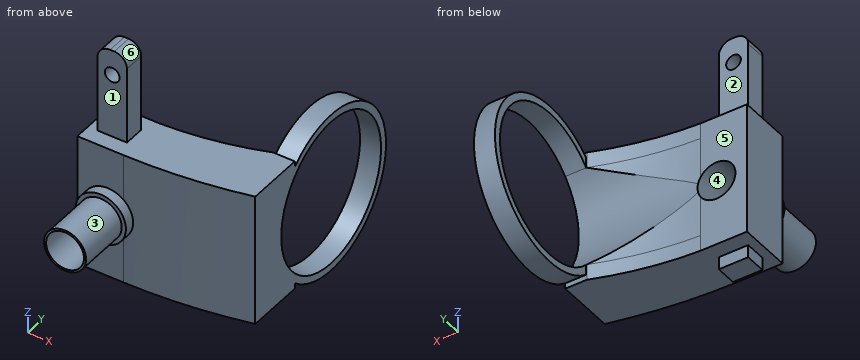
from build123d import *

# Parameters (mm, degrees)
BOSS_EXTRUDE1_DEPTH       = 48
SKETCH2_W                 = 14
SKETCH2_H                 = 10
BOSS_EXTRUDE2_DEPTH       = 50
CUT_EXTRUDE1_DEPTH        = 98
M8X1_0_TAPPED_HOLE1_D     = 7
M8X1_0_TAPPED_HOLE1_DEPTH = 10
M8X1_0_TAPPED_HOLE1_TIP   = 2.103012167
FILLET1_R                 = 6
SKETCH7_R                 = 38.5
SKETCH7_R_2               = 35
BOSS_EXTRUDE3_DEPTH       = 10
SKETCH8_R                 = 35
CUT_EXTRUDE2_DEPTH        = 90
BOSS_EXTRUDE4_DEPTH       = 5
BOSS_EXTRUDE4_DEPTH_BACK  = 10
SKETCH10_R                = 12
SKETCH10_R_2              = 9
BOSS_EXTRUDE5_START       = 25
SKETCH11_R                = 10
SKETCH11_R_2              = 9
BOSS_EXTRUDE5_DEPTH       = 25
SKETCH12_R                = 9
CUT_EXTRUDE3_DEPTH        = 42
BOSS_EXTRUDE6_DEPTH       = 7.5
BOSS_EXTRUDE7_START       = 7.5
BOSS_EXTRUDE7_DEPTH       = 7.5


with BuildPart() as part:
    # Sketch1 → Boss-Extrude1 (new body)
    with BuildSketch(Plane.XY):
        with BuildLine():
            Line((0, 0), (0, 25.00039893))
            Line((0, 25.00039893), (22, 25.00039893))
            ThreePointArc((22, 25.00039893), (51.667114877, 29.062120939), (80, 38.751440389))
            Line((80, 38.751440389), (80, 6.798665084))
            ThreePointArc((80, 6.798665084), (51.198552391, 1.705464917), (22, 0))
            Line((22, 0), (0, 0))
        make_face()
    extrude(amount=BOSS_EXTRUDE1_DEPTH)

    # Sketch2 → Boss-Extrude2 (add)
    with BuildSketch(Plane.XY.offset(48)):
        with Locations((11.5, 12.5)):
            Rectangle(SKETCH2_W, SKETCH2_H)
    boss_extrude2 = extrude(amount=BOSS_EXTRUDE2_DEPTH)

    # Mirror1: Boss-Extrude2 across plane
    add(boss_extrude2.mirror(Plane.XY.offset(24)))

    # Sketch3 → Cut-Extrude1 (cut)
    with BuildSketch(Plane(origin=(0, 0, 0), x_dir=(1, 0, 0), z_dir=(0, 1, 0))):
        Polygon((32.759036304, 13.5), (11.5, 13.5), (-23.123003772, 13.5), (-23.123003772, 84.867154232), (32.759036304, 84.867154232), align=None)
    extrude(amount=CUT_EXTRUDE1_DEPTH, mode=Mode.SUBTRACT)

    # M8x1.0 Tapped Hole1
    with Locations(Plane(origin=(11.5, 17.5, 86), x_dir=(0, 0, 1), z_dir=(0, 1, 0))):
        with Locations((0, 0)):
            Hole(M8X1_0_TAPPED_HOLE1_D / 2, depth=M8X1_0_TAPPED_HOLE1_DEPTH)
            with Locations((0, 0, -(M8X1_0_TAPPED_HOLE1_DEPTH + M8X1_0_TAPPED_HOLE1_TIP / 2))):  # 118° drill point
                Cone(0, M8X1_0_TAPPED_HOLE1_D / 2, M8X1_0_TAPPED_HOLE1_TIP, mode=Mode.SUBTRACT)

    # Fillet1
    fillet1_edges = [part.edges().sort_by_distance(p)[0] for p in [
        (18.5, 12.5, 98),
        (4.5, 12.5, 98),
    ]]
    fillet(fillet1_edges, radius=FILLET1_R)

    # Sketch7 → Boss-Extrude3 (add)
    with BuildSketch(Plane.ZY.offset(-80)):
        with Locations((24, 60.00039893)):
            Circle(SKETCH7_R)
        with Locations((24, 60.00039893)):
            Circle(SKETCH7_R_2, mode=Mode.SUBTRACT)
    extrude(amount=BOSS_EXTRUDE3_DEPTH)

    # Sketch8 → Cut-Extrude2 (cut)
    with BuildSketch(Plane.ZY.offset(-80)):
        with Locations(Location((24, 60.00039893, 0), (0, 0, 226.708192407))):
            Circle(SKETCH8_R)
    extrude(amount=CUT_EXTRUDE2_DEPTH, mode=Mode.SUBTRACT)

    # Sketch10 → Boss-Extrude4 (add, two sides: drawn at the far end of the back side and taken through both)
    with BuildSketch(Plane.XZ.offset(-BOSS_EXTRUDE4_DEPTH_BACK)):
        with Locations((14.5, 24)):
            Circle(SKETCH10_R)
        with Locations((14.5, 24)):
            Circle(SKETCH10_R_2, mode=Mode.SUBTRACT)
    extrude(amount=BOSS_EXTRUDE4_DEPTH + BOSS_EXTRUDE4_DEPTH_BACK)

    # Sketch11 → Boss-Extrude5 (add)
    with BuildSketch(Plane.XZ.offset(5).offset(BOSS_EXTRUDE5_START)):
        with Locations((14.5, 24)):
            Circle(SKETCH11_R)
        with Locations((14.5, 24)):
            Circle(SKETCH11_R_2, mode=Mode.SUBTRACT)
    extrude(amount=-BOSS_EXTRUDE5_DEPTH)

    # Sketch12 → Cut-Extrude3 (cut)
    with BuildSketch(Plane(origin=(0, 0, 0), x_dir=(-1, 0, 0), z_dir=(0, -1, 0))):
        with Locations(Location((-14.5, -24, 0), (0, 0, 180))):
            Circle(SKETCH12_R)
    extrude(amount=-CUT_EXTRUDE3_DEPTH, mode=Mode.SUBTRACT)

    # Sketch13 → Boss-Extrude6 (add)
    with BuildSketch(Plane.XY.offset(48)):
        with BuildLine():
            Line((0, 25.00039893), (0, 0))
            Line((0, 0), (22, 0))
            ThreePointArc((22, 0), (51.198552391, 1.705464917), (80, 6.798665084))
            Line((80, 6.798665084), (80, 29.896412483))
            Line((80, 29.896412483), (80, 34.524920524))
            Line((80, 34.524920524), (70, 34.524920524))
            Line((70, 34.524920524), (69.729925021, 34.524920524))
            ThreePointArc((69.729925021, 34.524920524), (46.24106465, 27.877911315), (22, 25.00039893))
            Line((22, 25.00039893), (0, 25.00039893))
        make_face()
    extrude(amount=BOSS_EXTRUDE6_DEPTH)

    # Sketch14 → Boss-Extrude7 (add)
    with BuildSketch(Plane(origin=(0, 0, 0), x_dir=(-1, 0, 0), z_dir=(0, 0, -1)).offset(BOSS_EXTRUDE7_START)):
        with BuildLine():
            Line((-80, 29.896412483), (-80, 6.798665084))
            ThreePointArc((-80, 6.798665084), (-51.198552391, 1.705464917), (-22, 0))
            Line((-22, 0), (0, 0))
            Line((0, 0), (0, 25.00039893))
            Line((0, 25.00039893), (-22, 25.00039893))
            ThreePointArc((-22, 25.00039893), (-46.24106465, 27.877911315), (-69.729925021, 34.524920524))
            Line((-69.729925021, 34.524920524), (-70, 34.524920524))
            Line((-70, 34.524920524), (-80, 34.524920524))
            Line((-80, 34.524920524), (-80, 29.896412483))
        make_face()
    extrude(amount=-BOSS_EXTRUDE7_DEPTH)


solid = part.part
Geometry: final body of the model. Coordinates: model frame, mm. Face numbers are marked on the shaded views. A direction names the side the tool comes from. Give positions to 0.01 mm unless a question says otherwise; leave off trailing zeros. Write each loop counter-clockwise with the first axis right and the second up, starting at its lowest first coordinate (ties: lowest second). Pieces come first, ordered by that corner, then holes. Notation, with made-up numbers: (79, 28) -> (87, 28) arc R27 ccw to (87, 56) -> close; hole circle Ø9 at (82, -24). An arc over 180 degrees is marked (long way). Answer as a JSON object with one key per item and string values.
1. Mould query, pull axis X, two halves, no side actions, for the marked faces 4, 5 and 6. Classes: pulls with the +X half, pulls with the -X half, needs draft (parallel to the pull), parting line crosses it, or undercut.
Ans:
{"face 4": "undercut", "face 5": "needs draft", "face 6": "pulls with the +X half"}
2. Access query for the marked faces 1, 2 and 3. Directions: +Z, -Z, +X, -X, +Y, -Y. A direction counts if a zero-diameter tool reaches every point of the face in a straight line with its end or side. Return the directions, or none.
Ans:
{"face 1": "+Z, +X, -X, -Y", "face 2": "+Z, +X, -X, +Y", "face 3": "-Y"}
3. Cut plane A-A on z = 24. Output: boundary loops of the cut face in (x, y).
Ans:
{"outline": "(0, 0) -> (2.5, 0) -> (2.5, -5) -> (4.5, -5) -> (4.5, -30) -> (5.5, -30) -> (5.5, 25) -> (0, 25) -> close; (23.5, -30) -> (24.5, -30) -> (24.5, -5) -> (26.5, -5) -> (26.5, 0.04) arc R250.8 ccw to (80, 6.8) -> (80, 25) -> (23.5, 25) -> close; (70, 95) -> (80, 95) -> (80, 98.5) -> (70, 98.5) -> close"}
4. Cut plane D-D on x = 36. Output: boundary loops of the cut face in (y, z).
Ans:
{"outline": "(0.39, -7.5) -> (26.19, -7.5) -> (26.19, 14.96) arc R35 cw to (26.19, 33.04) -> (26.19, 55.5) -> (0.39, 55.5) -> close"}
5. Cut plane C-C on y = 11.5. Output: boundary loops of the cut face in (x, z).
Ans:
{"outline": "(0, -7.5) -> (4.5, -7.5) -> (4.5, -13.5) -> (18.5, -13.5) -> (18.5, -7.5) -> (80, -7.5) -> (80, 55.5) -> (18.5, 55.5) -> (18.5, 92) arc R6 ccw to (12.5, 98) -> (10.5, 98) arc R6 ccw to (4.5, 92) -> (4.5, 55.5) -> (0, 55.5) -> close; hole circle Ø18 at (14.5, 24); hole circle Ø7 at (11.5, 86)"}
6. Ray query, probe 1 along Z at (x, y) = (11.5, 10); probe 2 along X at (y, z) = (14, 86); probe 3 along Z at (x, y) = (14.5, -10.5). Return the intervals inside material, ascending. Write a range as from..to.
Ans:
{"probe 1": "z = -13.5..15.51, 32.49..82.5, 89.5..98", "probe 2": "x = 4.5..8, 15..18.5", "probe 3": "z = 14..15, 33..34"}
7. Contact query for flat-ended pins moving along their axis: pin 1 (1.5 mm diameter, centred on y = 7.5, z = 58, fed in from -X); pin 2 (5 mm diameter, centred on y = 11, z = -9, fed in from -X); pin 3 (8 mm diameter, centred on x = 13.5, y = 11.5, fed in from -Z); pin 4 (6.5 mm diameter, centred on x = 14.5, z = -11, fed in from +Y). Output: stop coordinate, or through.
Ans:
{"pin 1": "stops at x = 4.5", "pin 2": "stops at x = 0", "pin 3": "stops at z = -13.5", "pin 4": "stops at y = 17.5"}
8. Cut plane B-B on z = 86. Output: boundary loops of the cut face in (x, y).
Ans:
{"outline": "(4.5, 7.5) -> (8, 7.5) -> (8, 17.5) -> (4.5, 17.5) -> close; (15, 7.5) -> (18.5, 7.5) -> (18.5, 17.5) -> (15, 17.5) -> close"}
